from build123d import *

# Parameters (mm, degrees)
F0_W     = 2.5
F0_H     = 3
F1_DEPTH = 5
F0_R     = 1.25
F2_DEPTH = 2
F3_DEPTH = 10
F0_W_2   = 3.75
F4_DEPTH = 5


with BuildPart() as f1:
    # F0 (on Front) → F1 (new body)
    with BuildSketch(Plane.XZ):
        with Locations((0, 14.5)):
            Rectangle(F0_W, F0_H)
    extrude(amount=F1_DEPTH)



with BuildPart() as f2:
    # F0 (on Front) → F2 (new body)
    with BuildSketch(Plane.XZ):
        with BuildLine():
            Line((-7.5, -8.5), (7.5, -8.5))
            ThreePointArc((7.5, -8.5), (8.2071067812, -8.2071067812), (8.5, -7.5))
            Line((8.5, -7.5), (8.5, 7.5))
            ThreePointArc((8.5, 7.5), (8.2071067812, 8.2071067812), (7.5, 8.5))
            Line((7.5, 8.5), (-7.5, 8.5))
            ThreePointArc((-7.5, 8.5), (-8.2071067812, 8.2071067812), (-8.5, 7.5))
            Line((-8.5, 7.5), (-8.5, -7.5))
            ThreePointArc((-8.5, -7.5), (-8.2071067812, -8.2071067812), (-7.5, -8.5))
        make_face()
        with Locations((0, -3.5)):
            Circle(F0_R, mode=Mode.SUBTRACT)
        with Locations((0, 3.5)):
            Circle(F0_R, mode=Mode.SUBTRACT)
    extrude(amount=F2_DEPTH)

    # F0 (on Front) → F3 (join)
    with BuildSketch(Plane.XZ):
        with BuildLine():
            Line((5, 10), (1.25, 10))
            Line((1.25, 10), (-1.25, 10))
            Line((-1.25, 10), (-5, 10))
            Line((-5, 10), (-9, 10))
            ThreePointArc((-9, 10), (-9.7071067812, 9.7071067812), (-10, 9))
            Line((-10, 9), (-10, -9))
            ThreePointArc((-10, -9), (-9.7071067812, -9.7071067812), (-9, -10))
            Line((-9, -10), (9, -10))
            ThreePointArc((9, -10), (9.7071067812, -9.7071067812), (10, -9))
            Line((10, -9), (10, 9))
            ThreePointArc((10, 9), (9.7071067812, 9.7071067812), (9, 10))
            Line((9, 10), (5, 10))
        make_face()
        with BuildLine():
            ThreePointArc((8.5, -7.5), (8.2071067812, -8.2071067812), (7.5, -8.5))
            Line((7.5, -8.5), (-7.5, -8.5))
            ThreePointArc((-7.5, -8.5), (-8.2071067812, -8.2071067812), (-8.5, -7.5))
            Line((-8.5, -7.5), (-8.5, 7.5))
            ThreePointArc((-8.5, 7.5), (-8.2071067812, 8.2071067812), (-7.5, 8.5))
            Line((-7.5, 8.5), (7.5, 8.5))
            ThreePointArc((7.5, 8.5), (8.2071067812, 8.2071067812), (8.5, 7.5))
            Line((8.5, 7.5), (8.5, -7.5))
        make_face(mode=Mode.SUBTRACT)
    extrude(amount=F3_DEPTH)


with BuildPart() as f1_1:
    add(f1.part)

    add(f2.part)  # F4 merges F2
    # F0 (on Front) → F4 (join)
    with BuildSketch(Plane.XZ):
        with Locations((-3.125, 11.5)):
            Rectangle(F0_W_2, F0_H)
        with Locations((0, 11.5)):
            Rectangle(F0_W, F0_H)
        with Locations((3.125, 11.5)):
            Rectangle(F0_W_2, F0_H)
    extrude(amount=F4_DEPTH)


solid = f1_1.part
Read the model definition and answer for the solid it produces. Units are mm, in the model's axes. A direction names the side the tool comes from. Coordinates: 2 decimals unless noted, no trailing zeros. Loops run counter-clockwise (first coordinate to the right, second up) from the corner with the lowest first, then second, coordinate; pieces in that order, holes last. Notation, with made-up numbers: (37.25, 21.5) -> (52.25, 21.5) arc R24 ccw to (52.25, 31.5) -> close; hole circle Ø2 at (6, 19). An arc over 180 degrees is marked (long way). Write item = value, one per line. Start each with the question number.
1) The part is cut by section D-D, the plane y = -1. Determine the outline of the cut face in (x, z), plus the area to 3 significant figures.
2) For faces 4 (the face through (0, -5, 12)), 5 (the face through (-5, -2, 11)), 6 (the face through (1.25, -2, 14)), 7 (the face through (-8.199, -5.944, -8.215)), 8 (the face through (-0.27, -0.99, -4.72)), determine the directions among +Z, -Z, +X, -X, +Y, -Y from which every point of the face is accessible in a straight line to the end or side of a thin tool.
3) The part is cut by section A-A, the plane x = -0.75. Determine the outline of the cut face in (y, z).
4) The part is cut by section C-C, the plane y = -3.5. Determine the outline of the cut face in (x, z).
5) The mould has two halves that part along X. Classify faces 1 (the face through (-9, -10, 0)), 2 (the face through (5, -2, 11)), 3 (the face through (8.199, -5.944, 8.215)): pulls with the +X half, pulls with the -X half, needs draft (parallel to the pull), parting line crosses it, or undercut.
6) The part is cut by section B-B, the plane z = -3.5. Determine the outline of the cut face in (x, y), plus the area to 3 significant figures.
7) Given P1, Ø1, axis at x = -6.5, y = -8, coming from the +Z side; P2, Ø1.5, axis at y = -2, z = 11.5, coming from the +X side; P3, Ø2.5, axis at y = -3, z = 15, coming from the +X side, each flat-ended and moving along its own axis, determine where each tip first touches the part or whether it passes through.
8) Find the intervals of material crossed by L1, parallel to Z at x = 0, y = -0.6; L2, parallel to Z at x = 7, y = -7, in increasing order. Write a range as from..to.
Result:
q1.outline = (-10, -9) arc R1 ccw to (-9, -10) -> (9, -10) arc R1 ccw to (10, -9) -> (10, 9) arc R1 ccw to (9, 10) -> (5, 10) -> (5, 13) -> (1.25, 13) -> (1.25, 16) -> (-1.25, 16) -> (-1.25, 13) -> (-5, 13) -> (-5, 10) -> (-9, 10) arc R1 ccw to (-10, 9) -> close; hole circle Ø2.5 at (0, -3.5); hole circle Ø2.5 at (0, 3.5)
q1.area = 427 mm²
q2.face_4 = +Z, +X, -X, -Y
q2.face_5 = +Z, -X, +Y, -Y
q2.face_6 = +Z, +X, +Y, -Y
q2.face_7 = -Y
q2.face_8 = +Y, -Y
q3.outline = (-10, -10) -> (0, -10) -> (0, -4.5) -> (-2, -4.5) -> (-2, -8.5) -> (-10, -8.5) -> close; (-10, 8.5) -> (-2, 8.5) -> (-2, 4.5) -> (0, 4.5) -> (0, 16) -> (-5, 16) -> (-5, 10) -> (-10, 10) -> close; (-2, -2.5) -> (0, -2.5) -> (0, 2.5) -> (-2, 2.5) -> close
q4.outline = (-10, -9) arc R1 ccw to (-9, -10) -> (9, -10) arc R1 ccw to (10, -9) -> (10, 9) arc R1 ccw to (9, 10) -> (5, 10) -> (5, 13) -> (1.25, 13) -> (1.25, 16) -> (-1.25, 16) -> (-1.25, 13) -> (-5, 13) -> (-5, 10) -> (-9, 10) arc R1 ccw to (-10, 9) -> close; hole (-8.5, -7.5) arc R1 ccw to (-7.5, -8.5) -> (7.5, -8.5) arc R1 ccw to (8.5, -7.5) -> (8.5, 7.5) arc R1 ccw to (7.5, 8.5) -> (-7.5, 8.5) arc R1 ccw to (-8.5, 7.5) -> close
q5.face_1 = needs draft
q5.face_2 = pulls with the +X half
q5.face_3 = undercut
q6.outline = (-10, -10) -> (-8.5, -10) -> (-8.5, -2) -> (-1.25, -2) -> (-1.25, 0) -> (-10, 0) -> close; (1.25, -2) -> (8.5, -2) -> (8.5, -10) -> (10, -10) -> (10, 0) -> (1.25, 0) -> close
q6.area = 59.0 mm²
q7.P1 = 10
q7.P2 = 5
q7.P3 = 1.25
q8.L1 = -10..-4.75, -2.25..2.25, 4.75..16
q8.L2 = -10..-8.5, 8.5..10
